```python
from build123d import *

# Parameters (mm, degrees)
F0_W     = 82.55
F0_H     = 76.2
F1_DEPTH = 3.175
F2_W     = 38.1
F2_H     = 38.1
F3_DEPTH = 3.175


with BuildPart() as f1:
    # F0 (on Top) → F1 (new body)
    with BuildSketch(Plane.XY):
        Rectangle(F0_W, F0_H)
    extrude(amount=F1_DEPTH)

    # F2 (on face) → F3 (cut)
    with BuildSketch(Plane(origin=(0, 0, 0), x_dir=(1, 0, 0), z_dir=(0, 0, -1))):
        Rectangle(F2_W, F2_H)
    extrude(amount=-F3_DEPTH, mode=Mode.SUBTRACT)


solid = f1.part
```
Geometry: final body of the model. Coordinates: model frame, mm. A direction names the side the tool comes from. Coordinates: 2 decimals unless noted, no trailing zeros. Write each loop counter-clockwise with the first axis right and the second up, starting at its lowest first coordinate (ties: lowest second). Pieces come first, ordered by that corner, then holes. Notation, with made-up numbers: M 80,17.25 L 89,17.25 A12 cw 89,23.25 Z; hole C -22,-28.5 d7. An arc over 180 degrees is marked long. Answer as CSV lines item,"result". Start each with the question number.
Q1. Reachability of faces 1 (the flat face through (0, 19.05, 2)), 2 (the flat face through (-1, 26, 3.175)) from +Z, -Z, +X, -X, +Y, -Y: full face, straight path, thin tool, end or side. Return the list, or none.
Q2. Cut plane B-B on z = 1. Return the cut outline in (x, y) (3 decimals).
Q3. Line query: line 1 (Y direction, x = -13.5, z = 2.2); line 2 (X direction, y = -11, z = 2.5) (3 decimals). Output: solid intervals per line, ascending. Write a range as from..to.
Q4. Mould query, pull axis Y, two halves, no side actions, for faces 3 (the flat face through (-1, -38.1, 2)), 4 (the flat face through (-1, 38.1, 2)), 5 (the flat face through (0, -19.05, 2)), 6 (the flat face through (-19.05, 0, 2)). Classes: released by +Y, released by -Y, zero draft, split by the parting line, or undercut.
Q5. Cut plane C-C on y = -18. Return the cut outline in (x, z) (3 decimals), then the cut area to 3 significant figures.
Q6. Cut plane A-A on x = -5.5. Return the cut outline in (y, z) (3 decimals), then the cut area to 3 significant figures.
Findings below:
1,face 1,"+Z, -Z"
1,face 2,"+Z, +X, -X, +Y, -Y"
2,outline,"M -41.275,-38.1 L 41.275,-38.1 L 41.275,38.1 L -41.275,38.1 Z; hole M -19.05,-19.05 L 19.05,-19.05 L 19.05,19.05 L -19.05,19.05 Z"
3,line 1,"y = -38.1..-19.05, 19.05..38.1"
3,line 2,"x = -41.275..-19.05, 19.05..41.275"
4,face 3,"released by -Y"
4,face 4,"released by +Y"
4,face 5,"undercut"
4,face 6,"undercut"
5,outline,"M -41.275,0 L -19.05,0 L -19.05,3.175 L -41.275,3.175 Z; M 19.05,0 L 41.275,0 L 41.275,3.175 L 19.05,3.175 Z"
5,area,"141 mm2"
6,outline,"M -38.1,0 L -19.05,0 L -19.05,3.175 L -38.1,3.175 Z; M 19.05,0 L 38.1,0 L 38.1,3.175 L 19.05,3.175 Z"
6,area,"121 mm2"
